Input: dimensioned drawing with shaded views. Units: mm. Origin: part minimum x, y, z. Coordinates: 2 decimals unless noted, no trailing zeros. Order: outer loops, then holes, each group sorted by start corner. A loop starts at its lowest first (then second) coordinate and runs counter-clockwise, first axis right, second up. Notation, with made-up numbers: (63.5, 85) -> (76.5, 85) arc R24 ccw to (76.5, 99) -> close; hole circle Ø4 at (16, 60.25). An arc over 180 degrees is marked (long way). Answer as CSV lines item,"result".
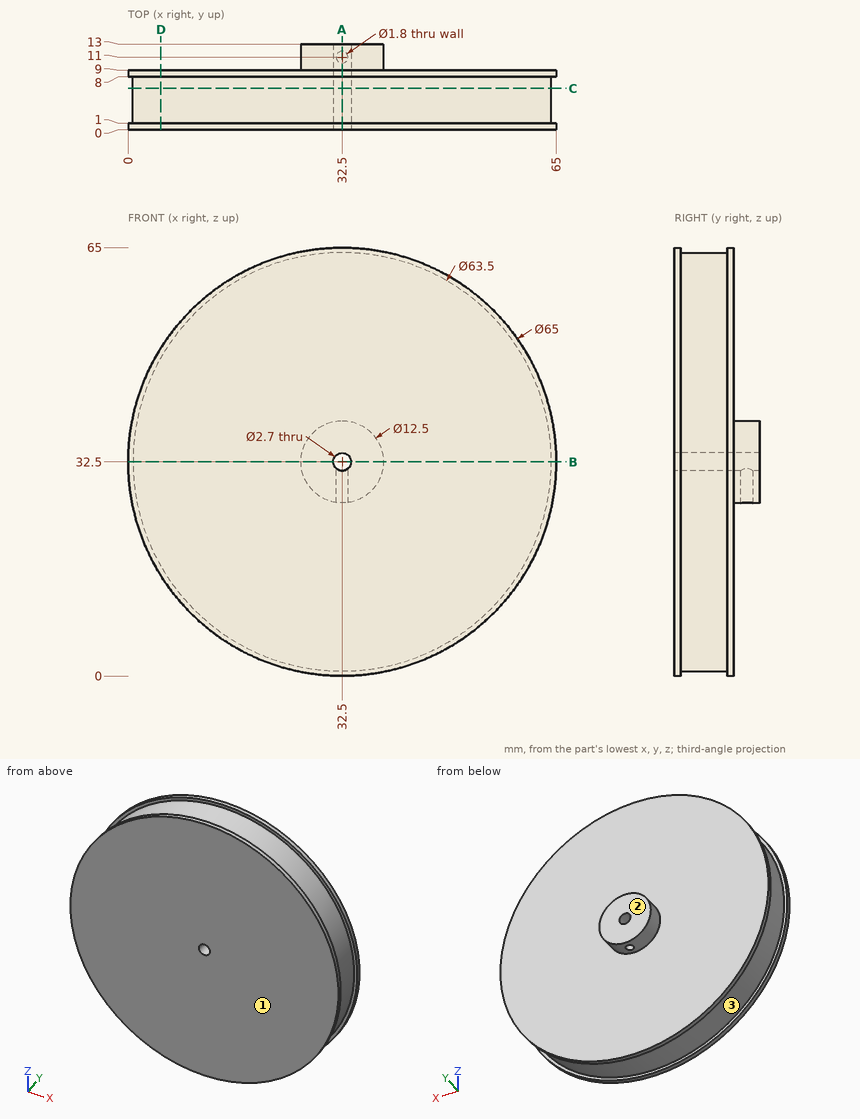
1. Cut plane A-A (x = 32.5). Return the cut outline in (y, z), plus the area to 3 significant figures.
Findings:
outline,"(0, 0) -> (1, 0) -> (1, 0.75) -> (8, 0.75) -> (8, 0) -> (9, 0) -> (9, 26.25) -> (10.1, 26.25) -> (10.1, 31.15) -> (0, 31.15) -> close; (0, 33.85) -> (13, 33.85) -> (13, 38.75) -> (9, 38.75) -> (9, 65) -> (8, 65) -> (8, 64.25) -> (1, 64.25) -> (1, 65) -> (0, 65) -> close; (11.9, 26.25) -> (13, 26.25) -> (13, 31.15) -> (11.9, 31.15) -> close"
area,"581 mm2"
2. Mould query, pull axis Y, two halves, no side actions, for the marked faces 1, 2 and 3. Classes: released by +Y, released by -Y, zero draft, split by the parting line, or undercut.
Findings:
face 1,"released by -Y"
face 2,"released by +Y"
face 3,"undercut"
3. Ray query, line 1 along X through (y, z) = (6.25, 32.5); line 2 along Y through (x, z) = (25, 33.5). Return the intervals inside material, ascending.
Findings:
line 1,"x = 0.75 to 31.15, 33.85 to 64.25"
line 2,"y = 0 to 9"
4. Cut plane C-C (y = 6.25). Return the cut outline in (x, z).
Findings:
outline,"circle Ø63.5 at (32.5, 32.5); hole circle Ø2.7 at (32.5, 32.5)"
5. Cut plane D-D (x = 5). Return the cut outline in (y, z), plus the area to 3 significant figures.
Findings:
outline,"(0, 15.18) -> (1, 15.18) -> (1, 16.63) -> (8, 16.63) -> (8, 15.18) -> (9, 15.18) -> (9, 49.82) -> (8, 49.82) -> (8, 48.37) -> (1, 48.37) -> (1, 49.82) -> (0, 49.82) -> close"
area,"291 mm2"
6. Contact query for flat-ended pins moving along their axis: pin 1 (2.5 mm diameter, centred on x = 32.5, z = 32.5, fed in from +Y); pin 2 (4 mm diameter, centred on x = 12, y = 10, fed in from +Z); pin 3 (4 mm diameter, centred on x = 47.5, y = 7, fed in from -Z); pin 4 (1.5 mm diameter, centred on y = 8.5, z = 33, fed in from -X). Output: stop coordinate, or through.
Findings:
pin 1,"passes through"
pin 2,"stops at z = 59.03"
pin 3,"stops at z = 2.83"
pin 4,"stops at x = 0"
7. Cut plane B-B (z = 32.5). Return the cut outline in (x, y), plus the area to 3 significant figures.
Findings:
outline,"(0, 0) -> (31.15, 0) -> (31.15, 13) -> (26.25, 13) -> (26.25, 9) -> (0, 9) -> (0, 8) -> (0.75, 8) -> (0.75, 1) -> (0, 1) -> close; (33.85, 0) -> (65, 0) -> (65, 1) -> (64.25, 1) -> (64.25, 8) -> (65, 8) -> (65, 9) -> (38.75, 9) -> (38.75, 13) -> (33.85, 13) -> close"
area,"589 mm2"
